Can you work these out from the model? Positions are in its coordinate system, mm. A direction names the side the tool comes from. Coordinates: 2 decimals unless noted, no trailing zeros. Write each loop counter-clockwise with the first axis right and the second up, starting at its lowest first coordinate (ties: lowest second). Pieces come first, ordered by that corner, then holes. Notation, with made-up numbers: (48.25, -31.75) - (52.25, -31.75) arc R16 ccw to (52.25, -12.75) - close; hole circle Ø6 at (78.5, -30). An arc over 180 degrees is marked (long way). Use one line per item in the form item = value. Start each with the question number.
(1) Thinking about a two-plate mould opening in Z: for faces 1 (the face through (4.521, 44.957, 64.651)), 2 (the face through (44.063, 75.893, 52.082)), 3 (the face through (43, 44, 56.15)), 4 (the face through (11, 6, 35)), which applies, pulls with the +Z half, pulls with the -Z half, needs draft (parallel to the pull), parting line crosses it, or undercut?
(2) For pin 1 Ø8 at (x, y) = (46.5, 34) entering from -Z; pin 2 Ø11 at (y, z) = (40, 62.5) entering from +X; pin 3 Ø4.5 at (y, z) = (40, 6) entering from +X; pin 4 Ø8.5 at (x, z) = (42, 50.5) entering from -Y, each with a flat end and sliding along its axis, tell me the tip position at first contact or that it passes through.
(3) On a 3-axis mill with a long thin cutter (end or side, diameter ignored), from which of +Z, -Z, +X, -X, +Y, -Y can I reach the whole of each face in a straight line? I mean faces 5 (the face through (4.521, 44.957, 6.651)), 6 (the face through (36.35, 70, 35)), 7 (the face through (6, 44, 35)). Say none if no direction works.
(4) If we section it at C-C on z = 40: Please give me the cut outline in (x, y), then the cut area to 3 significant figures.
(5) If we section it at B-B on y = 40: Please give me the cut outline in (x, z), then the cut area to 3 significant figures.
(6) If I drill on probe 1 along Y at (x, z) = (4.7, 64); probe 2 along Z at (x, y) = (42, 76.5); probe 3 along Y at (x, z) = (1, 6), over which ranges is the centre line in solid material (lowest first)? Write a range as from..to.
(7) If we section it at A-A on z = 64: Please give me the cut outline in (x, y), then the cut area to 3 significant figures.
(8) If we section it at D-D on x = 12: Please give me the cut outline in (y, z), then the cut area to 3 significant figures.
```python
from build123d import *

# Parameters (mm, degrees)
ESTRUSIONE_ESTRUSIONE1_DEPTH                         = 70
TAGLIO_ESTRUSIONE2_DEPTH                             = 133.233968783
TAGLIO_ESTRUSIONE2_DEPTH_BACK                        = 13.85
TAGLIO_ESTRUSIONE3_DEPTH                             = 13.85
FORO_LAMATO_PER_BULLONE_M12_A_TESTA_ESAG_D           = 5.4
FORO_LAMATO_PER_BULLONE_M12_A_TESTA_ESAG_DEPTH       = 18.1
FORO_LAMATO_PER_BULLONE_M12_A_TESTA_ESAG_CBORE_D     = 10
FORO_LAMATO_PER_BULLONE_M12_A_TESTA_ESAG_CBORE_DEPTH = 3
FORO_LAMATO_PER_BULLONE_M12_A_TESTA_ESAG_TIP         = 1.622323671
SMUSSO1_SIZE                                         = 10
SMUSSO1_SIZE2                                        = 7.11916601
FORO_PER_VITE_M4_1_D                                 = 5.2
FORO_PER_VITE_M4_1_DEPTH                             = 8.1
FORO_PER_VITE_M4_1_TIP                               = 1.562237609


with BuildPart() as part:
    # Schizzo1 → Estrusione-Estrusione1 (new body)
    with BuildSketch(Plane.XY):
        Polygon((0, 0), (0, 46), (6, 46), (6, 36), (36.35, 60), (36.35, 80), (78.65, 80), (78.65, 55.203294303), (16.42833408, 6), (6, 6), (6, 0), align=None)
    extrude(amount=ESTRUSIONE_ESTRUSIONE1_DEPTH)

    # Schizzo3 → Taglio-Estrusione2 (cut, two sides: drawn at the far end of the back side and taken through both)
    with BuildSketch(Plane.XY.offset(70).offset(-TAGLIO_ESTRUSIONE2_DEPTH_BACK)):
        Polygon((6, 6), (6, 36), (36.35, 60), (36.35, 80), (78.65, 80), (78.65, 55.203294303), (16.42833408, 6), align=None)
    extrude(amount=TAGLIO_ESTRUSIONE2_DEPTH + TAGLIO_ESTRUSIONE2_DEPTH_BACK, mode=Mode.SUBTRACT)

    # Schizzo4 → Taglio-Estrusione3 (cut)
    with BuildSketch(Plane(origin=(0, 0, 0), x_dir=(-1, 0, 0), z_dir=(0, 0, -1))):
        Polygon((-36.35, 60), (-36.35, 80), (-78.65, 80), (-78.65, 55.203294303), (-16.42833408, 6), (-6, 6), (-6, 36), align=None)
    extrude(amount=-TAGLIO_ESTRUSIONE3_DEPTH, mode=Mode.SUBTRACT)

    # Foro lamato per Bullone M12 a testa esagonale (Classe superiore)-1
    with Locations(Plane(origin=(6, 0, 0), x_dir=(0, 0, -1), z_dir=(1, 0, 0))):
        with Locations((-64, 6), (-6, 6), (-6, 40), (-64, 40)):
            CounterBoreHole(FORO_LAMATO_PER_BULLONE_M12_A_TESTA_ESAG_D / 2, FORO_LAMATO_PER_BULLONE_M12_A_TESTA_ESAG_CBORE_D / 2, FORO_LAMATO_PER_BULLONE_M12_A_TESTA_ESAG_CBORE_DEPTH, depth=FORO_LAMATO_PER_BULLONE_M12_A_TESTA_ESAG_DEPTH)
            with Locations((0, 0, -(FORO_LAMATO_PER_BULLONE_M12_A_TESTA_ESAG_DEPTH + FORO_LAMATO_PER_BULLONE_M12_A_TESTA_ESAG_TIP / 2))):  # 118° drill point
                Cone(0, FORO_LAMATO_PER_BULLONE_M12_A_TESTA_ESAG_D / 2, FORO_LAMATO_PER_BULLONE_M12_A_TESTA_ESAG_TIP, mode=Mode.SUBTRACT)

    # Smusso1
    smusso1_edges = [part.edges().sort_by_distance(p)[0] for p in [
        (6, 36, 35),
    ]]
    smusso1_side = [part.faces().sort_by_distance(p)[0] for p in [
        (21.175, 48, 35),
    ]]
    chamfer(smusso1_edges, length=SMUSSO1_SIZE, length2=SMUSSO1_SIZE2, reference=smusso1_side[0])

    # Foro per Vite M4-1
    with Locations(Plane(origin=(0, 80, 0), x_dir=(1, 0, 0), z_dir=(0, 1, 0))):
        with Locations((42, -19.5), (73, -19.5), (73, -50.5), (42, -50.5)):
            Hole(FORO_PER_VITE_M4_1_D / 2, depth=FORO_PER_VITE_M4_1_DEPTH)
            with Locations((0, 0, -(FORO_PER_VITE_M4_1_DEPTH + FORO_PER_VITE_M4_1_TIP / 2))):  # 118° drill point
                Cone(0, FORO_PER_VITE_M4_1_D / 2, FORO_PER_VITE_M4_1_TIP, mode=Mode.SUBTRACT)


solid = part.part
```
Reported:
q1.face_1 = undercut
q1.face_2 = undercut
q1.face_3 = pulls with the +Z half
q1.face_4 = needs draft
q2.pin_1 = 13.85
q2.pin_2 = 6
q2.pin_3 = through
q2.pin_4 = 22.86
q3.face_5 = +X
q3.face_6 = +Z, -Z, -X, +Y
q3.face_7 = none
q4.outline = (0, 0) - (6, 0) - (6, 6) - (16.43, 6) - (78.65, 55.2) - (78.65, 80) - (36.35, 80) - (36.35, 60) - (13.84, 42.2) - (6, 43.12) - (6, 46) - (0, 46) - close
q4.area = 3,180 mm2
q5.outline = (0, 0) - (6, 0) - (6, 1) - (3, 1) - (3, 3.3) - (0, 3.3) - close; (0, 8.7) - (3, 8.7) - (3, 11) - (6, 11) - (6, 13.85) - (59.42, 13.85) - (59.42, 56.15) - (6, 56.15) - (6, 59) - (3, 59) - (3, 61.3) - (0, 61.3) - close; (0, 66.7) - (3, 66.7) - (3, 69) - (6, 69) - (6, 70) - (0, 70) - close
q5.area = 2,590 mm2
q6.probe_1 = 0..1, 11..35, 45..46
q6.probe_2 = 13.85..16.9, 22.1..47.9, 53.1..56.15
q6.probe_3 = 0..3.3, 8.7..37.3, 42.7..46
q7.outline = (0, 0) - (6, 0) - (6, 1) - (3, 1) - (3, 3.3) - (0, 3.3) - close; (0, 8.7) - (3, 8.7) - (3, 11) - (6, 11) - (6, 35) - (3, 35) - (3, 37.3) - (0, 37.3) - close; (0, 42.7) - (3, 42.7) - (3, 45) - (6, 45) - (6, 46) - (0, 46) - close
q7.area = 184 mm2
q8.outline = (6, 13.85) - (42.42, 13.85) - (42.42, 56.15) - (6, 56.15) - close
q8.area = 1,540 mm2
